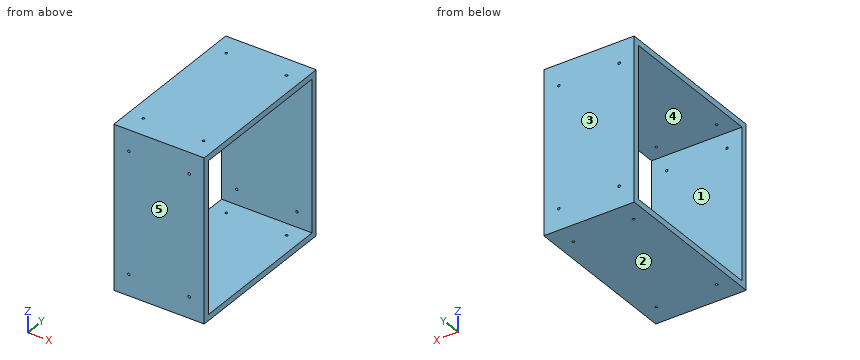
from build123d import *

# Parameters (mm, degrees)
EXTRUDE_1_DEPTH     = 300
SKETCH_2_R          = 4
CUT_EXTRUDE_1_DEPTH = 405.103947024


with BuildPart() as part:
    # 草图1 → 凸台-拉伸1 (new body)
    with BuildSketch(Plane(origin=(0, 0, 0), x_dir=(0, 0, -1), z_dir=(1, 0, 0))):
        Polygon((-250, 0), (-250, 250), (-270, 270), (-270, 0), align=None)
    extrude(amount=EXTRUDE_1_DEPTH)

    # 草图2 → 切除-拉伸1 (cut, through all)
    with BuildSketch(Plane(origin=(0, 0, 250), x_dir=(-1, 0, 0), z_dir=(0, 0, -1))):
        with Locations(Location((-250, 200, 0), (0, 0, 90))):
            Circle(SKETCH_2_R)
        with Locations(Location((-50, 200, 0), (0, 0, 90))):
            Circle(SKETCH_2_R)
    extrude(amount=-CUT_EXTRUDE_1_DEPTH, mode=Mode.SUBTRACT)

    # 镜向1: part across plane


with BuildPart() as part_1:
    add(part.part)
    add(part.part.mirror(Plane(origin=(300, 270, 270), x_dir=(0, 0.7071067811865485, 0.7071067811865466), z_dir=(0, -0.7071067811865466, 0.7071067811865485))))

    # 镜向2: part across plane


with BuildPart() as part_2:
    add(part_1.part)
    add(part_1.part.mirror(Plane(origin=(300, 250, 0), x_dir=(1, 0, 0), z_dir=(0, 0, 1))))

    # 镜向3: part across plane


with BuildPart() as part_3:
    add(part_2.part)
    add(part_2.part.mirror(Plane(origin=(300, 0, -250), x_dir=(0, 0, 1), z_dir=(0, 1, 0))))


solid = part_3.part
Read the model definition and answer for the solid it produces. Units are mm, in the model's axes. Face numbers are marked on the shaded views. A direction names the side the tool comes from. Coordinates: 2 decimals unless noted, no trailing zeros. Order: outer loops, then holes, each group sorted by start corner. A loop starts at its lowest first (then second) coordinate and runs counter-clockwise, first axis right, second up. Notation, with made-up numbers: (-15.5, -34) - (5.5, -34) arc R29 ccw to (5.5, -9) - close; hole circle Ø8 at (19, 66). An arc over 180 degrees is marked (long way). Use one line per item in the form item = value.
(1) Section A-A, the plane y = -101.5 is taken. Give the vertices of the cut face in (x, z), then the cut area to 3 significant figures.
Computed values:
outline = (0, -270) - (300, -270) - (300, -250) - (0, -250) - close; (0, 250) - (300, 250) - (300, 270) - (0, 270) - close
area = 12,000 mm²
(2) Straight lines are drawn through the part: L1, parallel to X at y = -257, z = -200; L2, parallel to Y at x = 68, z = 2. For each, find the intervals that lie inside material, in ascending order.
Computed values:
L1 = 0 to 46, 54 to 246, 254 to 300
L2 = -270 to -250, 250 to 270
(3) For a pull along Y with two mould halves and no side action, classify the marked faces 3, 4 and 5 as pulls with the +Y half, pulls with the -Y half, needs draft (parallel to the pull), parting line crosses it, or undercut.
Computed values:
face_3 = pulls with the +Y half
face_4 = undercut
face_5 = pulls with the -Y half
(4) Which of the six approach directions +Z, -Z, +X, -X, +Y, -Y give full straight-line access (tool end or side, diameter ignored) to the marked faces 1 and 2?
Computed values:
face_1 = +X, -X
face_2 = -Z, +X, -X, +Y, -Y
(5) Section C-C, the plane x = 187 is taken. Give the vertices of the cut face in (y, z), then the cut area to 3 significant figures.
Computed values:
outline = (-270, -270) - (270, -270) - (270, 270) - (-270, 270) - close; hole (-250, -250) - (250, -250) - (250, 250) - (-250, 250) - close
area = 41,600 mm²
